```python
from build123d import *

# Parameters (mm, degrees)
BOSS_EXTRUDE1_DEPTH = 12.7
SKETCH2_R           = 20.193
BOSS_EXTRUDE2_DEPTH = 21.336
SKETCH3_R           = 14.859
BOSS_EXTRUDE3_DEPTH = 4.572
SKETCH4_R           = 12.7
BOSS_EXTRUDE4_DEPTH = 12.7
BOSS_EXTRUDE4_TAPER = 2
SKETCH5_R           = 10.16
CUT_EXTRUDE1_DEPTH  = 61.347161428
FILLET1_R           = 2.54


with BuildPart() as part:
    # Sketch1 → Boss-Extrude1 (new body)
    with BuildSketch(Plane(origin=(0, 0, 0), x_dir=(1, 0, 0), z_dir=(0, 1, 0))):
        Polygon((15.211069479, -17.672003206), (22.909938452, 4.337170984), (7.698868973, 22.00917419), (-15.211069479, 17.672003206), (-22.909938452, -4.337170984), (-7.698868973, -22.00917419), align=None)
    extrude(amount=BOSS_EXTRUDE1_DEPTH)

    # Sketch2 → Boss-Extrude2 (add)
    with BuildSketch(Plane(origin=(0, 12.7, 0), x_dir=(1, 0, 0), z_dir=(0, 1, 0))):
        with Locations(Location((0, 0, 0), (0, 0, 100.720024221))):
            Circle(SKETCH2_R)
    extrude(amount=BOSS_EXTRUDE2_DEPTH)

    # Sketch3 → Boss-Extrude3 (add)
    with BuildSketch(Plane.XZ):
        with Locations(Location((0, 0, 0), (0, 0, 90))):
            Circle(SKETCH3_R)
    extrude(amount=BOSS_EXTRUDE3_DEPTH)

    # Sketch4 → Boss-Extrude4 (add)
    with BuildSketch(Plane.XZ.offset(4.572)):
        Circle(SKETCH4_R)
    extrude(amount=BOSS_EXTRUDE4_DEPTH, taper=BOSS_EXTRUDE4_TAPER)

    # Sketch5 → Cut-Extrude1 (cut, through all)
    with BuildSketch(Plane.XZ.offset(17.272)):
        with Locations(Location((0, 0, 0), (0, 0, 270))):
            Circle(SKETCH5_R)
    extrude(amount=-CUT_EXTRUDE1_DEPTH, mode=Mode.SUBTRACT)

    # Fillet1
    # the kernel refuses this fillet: 2.54 mm, written as the material it takes off along each edge
    with BuildSketch(Plane(origin=(-7.698868973, -3.666174209, 22.00917419), x_dir=(0.9825478481724581, 0, -0.18601001599825806), z_dir=(0, 1, 0)), Plane(origin=(-22.909938452, -3.666174209, 4.337170984), x_dir=(0.6523633232990701, 0, 0.7579063889519556), z_dir=(0, 1, 0)), Plane(origin=(15.211069479, -3.666174209, 17.672003206), x_dir=(0.3301845248733872, 0, -0.9439164049502137), z_dir=(0, 1, 0))) as fillet1_piece_1:
        with BuildLine():
            CenterArc((FILLET1_R * 0.57735026919, FILLET1_R), FILLET1_R, 210, 60)
            Line((-FILLET1_R * 0.288675134595, FILLET1_R * 0.5), (-FILLET1_R * 0.305995642671, FILLET1_R * 0.49))
            Line((-FILLET1_R * 0.305995642671, FILLET1_R * 0.49), (-FILLET1_R * 0.0115470053838, -FILLET1_R * 0.02))
            Line((-FILLET1_R * 0.0115470053838, -FILLET1_R * 0.02), (FILLET1_R * 0.57735026919, -FILLET1_R * 0.02))
            Line((FILLET1_R * 0.57735026919, -FILLET1_R * 0.02), (FILLET1_R * 0.57735026919, 0))
        make_face()
    extrude(amount=20.032348419, mode=Mode.SUBTRACT)
    with BuildSketch(Plane(origin=(-15.211069479, -3.666174209, -17.672003206), x_dir=(0.9825478481724584, 0, -0.18601001599825617), z_dir=(0, 1, 0)), Plane(origin=(7.698868973, -3.666174209, -22.00917419), x_dir=(0.6523633232990698, 0, 0.7579063889519558), z_dir=(0, 1, 0)), Plane(origin=(22.909938452, -3.666174209, -4.337170984), x_dir=(-0.33018452487338784, 0, 0.9439164049502133), z_dir=(0, 1, 0))) as fillet1_piece_2:
        with BuildLine():
            CenterArc((FILLET1_R * 0.57735026919, -FILLET1_R), FILLET1_R, 90, 60)
            Line((-FILLET1_R * 0.288675134595, -FILLET1_R * 0.5), (-FILLET1_R * 0.305995642671, -FILLET1_R * 0.49))
            Line((-FILLET1_R * 0.305995642671, -FILLET1_R * 0.49), (-FILLET1_R * 0.0115470053838, FILLET1_R * 0.02))
            Line((-FILLET1_R * 0.0115470053838, FILLET1_R * 0.02), (FILLET1_R * 0.57735026919, FILLET1_R * 0.02))
            Line((FILLET1_R * 0.57735026919, FILLET1_R * 0.02), (FILLET1_R * 0.57735026919, 0))
        make_face()
    extrude(amount=20.032348419, mode=Mode.SUBTRACT)
    with BuildSketch(Plane(origin=(0, -4.572, 0), x_dir=(0, 0, 1), z_dir=(1, 0, 0))) as fillet1_piece_3:
        with BuildLine():
            CenterArc((12.319, -2.511262432), FILLET1_R, 0, 81.373073441)
            Line((12.7, 0), (12.70762, 0.050225249))
            ThreePointArc((12.70762, 0.050225249), (13.7795, 0.0508), (14.859, 0.0508))
            Line((14.859, 0.0508), (14.9098, 0))
            Line((14.9098, 0), (14.9098, -2.511262432))
            Line((14.9098, -2.511262432), (14.859, -2.511262432))
        make_face()
    revolve(axis=Axis((0, -4.572, 0), (0, -1, 0)), mode=Mode.SUBTRACT)


solid = part.part
```
Read the model definition and answer for the solid it produces. Units are mm, in the model's axes. A direction names the side the tool comes from. Coordinates: 2 decimals unless noted, no trailing zeros. Loops run counter-clockwise (first coordinate to the right, second up) from the corner with the lowest first, then second, coordinate; pieces in that order, holes last.
(1) The part is cut by section C-C (y = -3.5). Determine the outline of the cut face in (x, z), and give its area (3 significant figures).
Solution:
outline: circle Ø28.82 at (0, 0); hole circle Ø20.32 at (0, 0)
area: 328 mm2
(2) The mould has two halves that part along Z. Classify faces 3 (the face through (7, 12.7, -20)), 4 (the face through (-3.616, 6.261, -19.867)), 5 (the face through (2.88, 23.219, 19.987)), 6 (the face through (10.074, 8.023, 1.323)): released by +Z, released by -Z, zero draft, split by the parting line, or undercut.
Solution:
face 3: zero draft
face 4: released by -Z
face 5: split by the parting line
face 6: undercut
(3) A tool of negligible diameter and unlimited length cuts with its end or side. For faces 1 (the face through (14, 12.7, 16)), 2 (the face through (7.59, 6.26, -21.63)), from which of +Z, -Z, +X, -X, +Y, -Y can it reach the whole face along a straight path? Write none if from no direction.
Solution:
face 1: +Z, +X, +Y
face 2: -Z, +Y, -Y
(4) The part is cut by section A-A (y = 12). Determine the outline of the cut face in (x, z).
Solution:
outline: (-22.43, 2.95) - (-15.7, -16.29) arc R2.54 ccw to (-13.77, -17.94) - (6.26, -21.74) arc R2.54 ccw to (8.66, -20.9) - (21.95, -5.45) arc R2.54 ccw to (22.43, -2.95) - (15.7, 16.29) arc R2.54 ccw to (13.77, 17.94) - (-6.26, 21.74) arc R2.54 ccw to (-8.66, 20.9) - (-21.95, 5.45) arc R2.54 ccw to start; hole circle Ø20.32 at (0, 0)
(5) Flat-ended cylindrical pins translate along their axes: pin 1 Ø4 at (x, y) = (2, 22) entering from -Z; pin 2 Ø8 at (x, z) = (12.5, 11.5) entering from -Y; pin 3 Ø6 at (y, z) = (-0.5, -8) entering from -X; pin 4 Ø10 at (x, z) = (-1, 9) entering from -Y. Find the tip coordinate at first contact, or state that the pin passes through.
Solution:
pin 1: stops at z = -20.19
pin 2: stops at y = -4.51
pin 3: stops at x = -19.63
pin 4: stops at y = -17.27
(6) Consider line 1 along X through (y, z) = (18, 0); line 2 along Y through (x, z) = (10.5, 18); line 3 along Z through (x, y) = (-0.5, 3.5). Determine where each line is inside the solid, lowest interval first.
Solution:
line 1: x = -20.19 to -10.16, 10.16 to 20.19
line 2: y = 0 to 12.7
line 3: z = -20.46 to -10.15, 10.15 to 20.65
(7) The part is cut by section B-B (x = 0). Determine the outline of the cut face in (y, z), and give its area (3 significant figures).
Solution:
outline: (-17.27, -12.26) - (-4.57, -12.7) arc R2.54 ccw to (-2.06, -14.86) - (0, -14.86) - (0, -20.55) - (12.7, -20.55) - (12.7, -20.19) - (34.04, -20.19) - (34.04, -10.16) - (-17.27, -10.16) - close; (-17.27, 10.16) - (34.04, 10.16) - (34.04, 20.19) - (12.7, 20.19) - (12.7, 20.55) - (0, 20.55) - (0, 14.86) - (-2.06, 14.86) arc R2.54 ccw to (-4.57, 12.7) - (-17.27, 12.26) - close
area: 791 mm2
